Read the model definition and answer for the solid it produces. Units are mm, in the model's axes. Face numbers are marked on the shaded views. A direction names the side the tool comes from. Coordinates: 2 decimals unless noted, no trailing zeros. Write each loop counter-clockwise with the first axis right and the second up, starting at its lowest first coordinate (ties: lowest second). Pieces come first, ordered by that corner, then holes. Notation, with made-up numbers: (-22.75, 66) -> (10.25, 66) arc R25 cw to (10.25, 93) -> close; hole circle Ø1 at (-7, -10). An arc over 180 degrees is marked (long way). Write item = value, one per line. Start each with the question number.
1) Section A-A (x = 0) is taken. Determine the outline of the cut face in (y, z), plus the area to 3 significant figures.
2) Section D-D (z = -14.5) is taken. Determine the outline of the cut face in (x, y).
3) Section B-B (z = 0) is taken. Determine the outline of the cut face in (x, y).
4) A tool of negligible diameter and unlimited length cuts with its end or side. For the marked faces 1, 2, 3, 4 and 5, from which of +Z, -Z, +X, -X, +Y, -Y can it reach the whole face along a straight path? Write none if from no direction.
5) Find the intervals of material crossed by line 1 along X through (y, z) = (-284.25, 0); line 2 along Z through (x, y) = (-7, -9.5); line 3 along Y through (x, z) = (-4, 11.5), in increasing order. Write a range as from..to.
6) Flat-ended cylindrical pins translate along their axes: pin 1 Ø1 at (x, z) = (15.5, -3.5) entering from -Y; pin 2 Ø8 at (x, z) = (0, 0) entering from -Y; pin 3 Ø10 at (y, z) = (-73.5, -2) entering from -X; pin 4 Ø8 at (x, z) = (2.5, -1) entering from -Y. Find the tip coordinate at first contact, or state that the pin passes through.
7) Section C-C (y = -42.5) is taken. Determine the outline of the cut face in (x, z).
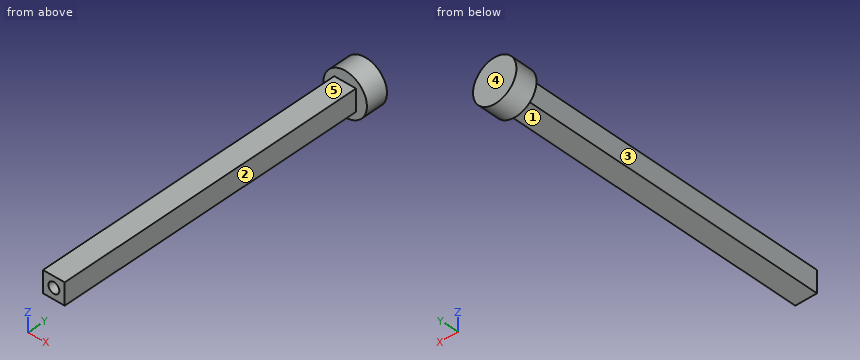
from build123d import *

# Parameters (mm, degrees)
SKETCH2_R           = 20
BOSS_EXTRUDE1_DEPTH = 20
SKETCH3_W           = 20
SKETCH3_H           = 20
BOSS_EXTRUDE2_DEPTH = 290
SKETCH4_R           = 5
CUT_EXTRUDE1_DEPTH  = 10


with BuildPart() as part:
    # Sketch2 → Boss-Extrude1 (new body)
    with BuildSketch(Plane(origin=(0, 0, 0), x_dir=(1, 0, 0), z_dir=(0, 1, 0))):
        with Locations(Location((0, 0, 0), (0, 0, 270))):
            Circle(SKETCH2_R)
    extrude(amount=BOSS_EXTRUDE1_DEPTH)

    # Sketch3 → Boss-Extrude2 (add)
    with BuildSketch(Plane.XZ):
        Rectangle(SKETCH3_W, SKETCH3_H)
    extrude(amount=BOSS_EXTRUDE2_DEPTH)

    # Sketch4 → Cut-Extrude1 (cut)
    with BuildSketch(Plane.XZ.offset(290)):
        with Locations(Location((0, 0, 0), (0, 0, 270))):
            Circle(SKETCH4_R)
    extrude(amount=-CUT_EXTRUDE1_DEPTH, mode=Mode.SUBTRACT)


solid = part.part
Answer key:
q1.outline = (-290, -10) -> (0, -10) -> (0, -20) -> (20, -20) -> (20, 20) -> (0, 20) -> (0, 10) -> (-290, 10) -> (-290, 5) -> (-280, 5) -> (-280, -5) -> (-290, -5) -> close
q1.area = 6,500 mm^2
q2.outline = (-13.77, 0) -> (13.77, 0) -> (13.77, 20) -> (-13.77, 20) -> close
q3.outline = (-20, 0) -> (-10, 0) -> (-10, -290) -> (-5, -290) -> (-5, -280) -> (5, -280) -> (5, -290) -> (10, -290) -> (10, 0) -> (20, 0) -> (20, 20) -> (-20, 20) -> close
q4.face_1 = -Z, +X, -X, -Y
q4.face_2 = +Z, -Z, +X, -Y
q4.face_3 = +Z, -Z, -X, -Y
q4.face_4 = +Z, -Z, +X, -X, +Y
q4.face_5 = +Z, +X, -X, -Y
q5.line_1 = -10..-5, 5..10
q5.line_2 = -10..10
q5.line_3 = 0..20
q6.pin_1 = 0
q6.pin_2 = -280
q6.pin_3 = -10
q6.pin_4 = -290
q7.outline = (-10, -10) -> (10, -10) -> (10, 10) -> (-10, 10) -> close
